Geometry: final body of the model. Coordinates: model frame, mm. A direction names the side the tool comes from. Give positions to 0.01 mm unless a question says otherwise; leave off trailing zeros. Write each loop counter-clockwise with the first axis right and the second up, starting at its lowest first coordinate (ties: lowest second). Pieces come first, ordered by that corner, then holes. Notation, with made-up numbers: (-14, 13.5) -> (-1, 13.5) arc R32 ccw to (-1, 47.5) -> close; hole circle Ø1 at (11, 59). An arc over 180 degrees is marked (long way). Answer as a JSON object with one key per item and string values.
from build123d import *

# Parameters (mm, degrees)
SKETCH1_R           = 12.5
BOSS_EXTRUDE1_DEPTH = 10
SKETCH2_R           = 15
BOSS_EXTRUDE2_DEPTH = 15
SKETCH3_R           = 12.5
CUT_EXTRUDE1_DEPTH  = 2


with BuildPart() as part:
    # Sketch1 → Boss-Extrude1 (new body)
    with BuildSketch(Plane(origin=(0, 0, 0), x_dir=(1, 0, 0), z_dir=(0, 1, 0))):
        Circle(SKETCH1_R)
    extrude(amount=BOSS_EXTRUDE1_DEPTH)

    # Sketch2 → Boss-Extrude2 (add)
    with BuildSketch(Plane(origin=(0, 10, 0), x_dir=(1, 0, 0), z_dir=(0, 1, 0))):
        Circle(SKETCH2_R)
    extrude(amount=BOSS_EXTRUDE2_DEPTH)

    # Sketch3 → Cut-Extrude1 (cut)
    with BuildSketch(Plane(origin=(0, 25, 0), x_dir=(1, 0, 0), z_dir=(0, 1, 0))):
        Circle(SKETCH3_R)
    extrude(amount=-CUT_EXTRUDE1_DEPTH, mode=Mode.SUBTRACT)


solid = part.part
Q1. First-contact query: P1, Ø1, axis at x = -6.5, y = 4, coming from the -Z side; P2, Ø3, axis at y = 15, z = -9, coming from the +X side; P3, Ø2, axis at y = 5, z = -7.5, coming from the +X side. Flat tips, straight axial feed; report the tip coordinate or a pass-through.
Values:
{"P1": "z = -10.97", "P2": "x = 12.99", "P3": "x = 10.68"}
Q2. Cut plane A-A (z = 0). Return the cut outline in (x, y), and give its area (3 significant figures).
Values:
{"outline": "(-15, 10) -> (-12.5, 10) -> (-12.5, 0) -> (12.5, 0) -> (12.5, 10) -> (15, 10) -> (15, 25) -> (12.5, 25) -> (12.5, 23) -> (-12.5, 23) -> (-12.5, 25) -> (-15, 25) -> close", "area": "650 mm²"}
Q3. Set-up query: faces 4 (the flat face through (-3.4, 25, -12.3)), 5 (the flat face through (-3.4, 10, -12.3)), 6 (the flat face through (0, 23, 0)). Return all of +Z, -Z, +X, -X, +Y, -Y with unobstructed straight access to the full face (end or side cutting, diameter ignored); none if empty.
Values:
{"face 4": "+Z, -Z, +X, -X, +Y", "face 5": "-Y", "face 6": "+Y"}
Q4. Cut plane C-C (y = 19). Return the cut outline in (x, z), and give its area (3 significant figures).
Values:
{"outline": "circle Ø30 at (0, 0)", "area": "707 mm²"}
Q5. Mould query, pull axis Z, two halves, no side actions, for faces 1 (the cylindrical face through (11.923, 24.014, -3.755)), 2 (the flat face through (0, 0, 0)), 3 (the cylindrical face through (-14.985, 17.395, -0.66)). Classes: pulls with the +Z half, pulls with the -Z half, needs draft (parallel to the pull), parting line crosses it, or undercut.
Values:
{"face 1": "undercut", "face 2": "needs draft", "face 3": "parting line crosses it"}
Q6. Material intervals for L1, parallel to X at y = 24.45, z = 0; L2, parallel to Y at x = 8.25, z = -5.5, sorted ascending. Write a range as from..to.
Values:
{"L1": "-15..-12.5, 12.5..15", "L2": "0..23"}
Q7. Cut plane D-D (y = 3.75). Return the cut outline in (x, z).
Values:
{"outline": "circle Ø25 at (0, 0)"}
Q8. Cut plane B-B (x = 0). Return the cut outline in (y, z).
Values:
{"outline": "(0, -12.5) -> (10, -12.5) -> (10, -15) -> (25, -15) -> (25, -12.5) -> (23, -12.5) -> (23, 12.5) -> (25, 12.5) -> (25, 15) -> (10, 15) -> (10, 12.5) -> (0, 12.5) -> close"}
